Could you check a few things on this model? Use its own coordinates, in mm. Round coordinates to 2 decimals unless told otherwise and drop trailing zeros. Write each loop counter-clockwise with the first axis right and the second up, starting at its lowest first coordinate (ties: lowest second). Pieces come first, ordered by that corner, then holes. Notation, with made-up numbers: M 9,64 L 65,64 A23 cw 65,82 Z; hole C 79.25,-38 d7. An arc over 180 degrees is marked long. One line per question, with ' | ' between items. Start each with the question number.
```python
from build123d import *


with BuildPart() as cone:
    # Cone → Cone (revolve)
    with BuildSketch(Plane.XZ):
        Polygon((0, 0), (40, 0), (0, 200), align=None)
    revolve(axis=Axis((0, 0, 0), (0, 0, 1)))


with BuildPart() as fusion:
    # Sphere001 → Sphere001 (revolve)
    with BuildSketch(Plane.XZ):
        with BuildLine():
            ThreePointArc((0, -50), (50, 0), (0, 50))
            Line((0, 50), (0, -50))
        make_face()
    revolve(axis=Axis((0, 0, 0), (0, 0, 1)))

    # Fusion: union Cone
    add(cone.part)


solid = fusion.part
```
1. I need wall thicknesses on line 1 along Z through (x, y) = (-3, -38); line 2 along Y through (x, z) = (-29.5, -34); line 3 along Y through (x, z) = (40.5, 18). Which ranges of each line are inside material? Lowest first, please. Write a range as from..to.
2. I'm going to push flat-ended pins straight in: P1, Ø5, axis at x = 11, y = 31.5, coming from the -Z side; P2, Ø5, axis at x = 32, y = -27.5, coming from the +Z side (3 decimals); P3, Ø12, axis at x = -4, z = 163, coming from the -Y side. Where does each tip first touch, or does it pass through?
3. Suppose I cut it at B-B (x = 42). Write out the boundary of the cut face in (y, z).
4. Suppose I cut it at A-A (z = 151). Write out the boundary of the cut face in (x, y), and give its area (3 significant figures).
Computed:
1) line 1: z = -32.36..32.36 | line 2: y = -21.77..21.77 | line 3: y = -23.15..23.15
2) P1: stops at z = -39.34 | P2: stops at z = 30.405 | P3: stops at y = -8.38
3) outline: C 0,0 d54.26
4) outline: C 0,0 d19.6 | area: 302 mm²
